The listing builds one solid part. Answer for the finished solid, in the listing's coordinates (mm). A direction names the side the tool comes from. Give positions to 0.01 mm unless a question says otherwise; leave off trailing zeros. Write each loop counter-clockwise with the first axis right and the second up, starting at its lowest first coordinate (ties: lowest second). Pieces come first, ordered by that corner, then holes. Notation, with made-up numbers: M 61.25,26 L 100.25,26 A22 ccw 100.25,62 Z; hole C -26.5,-36.5 d8. An arc over 180 degrees is marked long. Return JSON: item names as keys, results as strings.
from build123d import *

# Parameters (mm, degrees)
SKETCH1_R               = 2.25
BOSS_EXTRUDE1_DEPTH     = 7.5
CUT_EXTRUDE1_START      = 7.5
SKETCH1_3_R             = 6.52
CUT_EXTRUDE1_DEPTH      = 5
CUT_EXTRUDE2_START      = -7.5
SKETCH1_4_R             = 6.52
CUT_EXTRUDE2_DEPTH      = 5
SKETCH2_R               = 14.4
BOSS_EXTRUDE2_DEPTH     = 19
CUT_EXTRUDE3_DEPTH      = 51.395634732
CUT_EXTRUDE3_DEPTH_BACK = 51.395634732
CUT_EXTRUDE4_DEPTH      = 7
CUT_EXTRUDE5_START      = -12
SKETCH2_5_R             = 11.4
CUT_EXTRUDE5_DEPTH      = 7
FILLET1_R               = 5
FILLET2_R               = 10
FILLET3_R               = 5


with BuildPart() as part:
    # Sketch1 → Boss-Extrude1 (new, symmetric)
    with BuildSketch(Plane.XY):
        Polygon((-9.5, 9), (9.5, 9), (9.5, -10.52), (-5.5, -25.52), (-30, -25.52), (-30, -6.52), (-9.5, -6.52), align=None)
        Circle(SKETCH1_R, mode=Mode.SUBTRACT)
    extrude(amount=BOSS_EXTRUDE1_DEPTH, both=True)

    # Sketch1<3> → Cut-Extrude1 (cut)
    with BuildSketch(Plane.XY.offset(CUT_EXTRUDE1_START)):
        Circle(SKETCH1_3_R)
    extrude(amount=-CUT_EXTRUDE1_DEPTH, mode=Mode.SUBTRACT)

    # Sketch1<4> → Cut-Extrude2 (cut)
    with BuildSketch(Plane.XY.offset(CUT_EXTRUDE2_START)):
        Circle(SKETCH1_4_R)
    extrude(amount=CUT_EXTRUDE2_DEPTH, mode=Mode.SUBTRACT)

    # Sketch2 → Boss-Extrude2 (add, through all)
    with BuildSketch(Plane(origin=(0, -6.52, 0), x_dir=(1, 0, 0), z_dir=(0, 1, 0))):
        with Locations((-30, 0)):
            Circle(SKETCH2_R)
    extrude(amount=-BOSS_EXTRUDE2_DEPTH)

    # Sketch2<3> → Cut-Extrude3 (cut, two sides: drawn at the far end of the back side and taken through both)
    with BuildSketch(Plane(origin=(0, -6.52, 0), x_dir=(1, 0, 0), z_dir=(0, 1, 0)).offset(-CUT_EXTRUDE3_DEPTH_BACK)):
        with BuildLine():
            ThreePointArc((-30, -4.25), (-26.99479618, -3.00520382), (-25.75, 0))
            ThreePointArc((-25.75, 0), (-26.99479618, 3.00520382), (-30, 4.25))
            Line((-30, 4.25), (-30, -4.25))
        make_face()
        with BuildLine():
            Line((-30, -4.25), (-30, 4.25))
            ThreePointArc((-30, 4.25), (-34.25, 0), (-30, -4.25))
        make_face()
    extrude(amount=CUT_EXTRUDE3_DEPTH + CUT_EXTRUDE3_DEPTH_BACK, mode=Mode.SUBTRACT)

    # Sketch2<4> → Cut-Extrude4 (cut)
    with BuildSketch(Plane(origin=(0, -6.52, 0), x_dir=(1, 0, 0), z_dir=(0, 1, 0))):
        with BuildLine():
            ThreePointArc((-21.414547187, -7.5), (-19.326805491, -4.005361278), (-18.6, 0))
            ThreePointArc((-18.6, 0), (-19.326805491, 4.005361278), (-21.414547187, 7.5))
            Line((-21.414547187, 7.5), (-30, 7.5))
            Line((-30, 7.5), (-30, 4.25))
            ThreePointArc((-30, 4.25), (-26.99479618, 3.00520382), (-25.75, 0))
            ThreePointArc((-25.75, 0), (-26.99479618, -3.00520382), (-30, -4.25))
            Line((-30, -4.25), (-30, -7.5))
            Line((-30, -7.5), (-21.414547187, -7.5))
        make_face()
        with BuildLine():
            Line((-30, 7.5), (-21.414547187, 7.5))
            ThreePointArc((-21.414547187, 7.5), (-41.4, 0), (-21.414547187, -7.5))
            Line((-21.414547187, -7.5), (-30, -7.5))
            Line((-30, -7.5), (-30, -4.25))
            ThreePointArc((-30, -4.25), (-34.25, 0), (-30, 4.25))
            Line((-30, 4.25), (-30, 7.5))
        make_face()
    extrude(amount=-CUT_EXTRUDE4_DEPTH, mode=Mode.SUBTRACT)

    # Sketch2<5> → Cut-Extrude5 (cut)
    with BuildSketch(Plane(origin=(0, -6.52, 0), x_dir=(1, 0, 0), z_dir=(0, 1, 0)).offset(CUT_EXTRUDE5_START)):
        with Locations(Location((-30, 0, 0), (0, 0, 270))):
            Circle(SKETCH2_5_R)
    extrude(amount=-CUT_EXTRUDE5_DEPTH, mode=Mode.SUBTRACT)

    # Fillet1
    fillet1_edges = [part.edges().sort_by_distance(p)[0] for p in [
        (-9.5, -6.52, 0),
        (-17.707319251, -16.02, -7.5),
        (-17.707319251, -16.02, 7.5),
    ]]
    fillet(fillet1_edges, radius=FILLET1_R)

    # Fillet2
    # the kernel refuses this fillet: 10 mm, written as the material it takes off along each edge
    with BuildSketch(Plane(origin=(-9.5, 9, -32.5), x_dir=(0, -1, 0), z_dir=(0, 0, 1))) as fillet2_piece_1:
        with BuildLine():
            CenterArc((FILLET2_R, FILLET2_R), FILLET2_R, 180, 90)
            Line((0, FILLET2_R), (0, 0))
            Line((0, 0), (FILLET2_R, 0))
        make_face()
    extrude(amount=65, mode=Mode.SUBTRACT)
    with BuildSketch(Plane(origin=(9.5, 9, 32.5), x_dir=(-1, 0, 0), z_dir=(0, 0, -1))) as fillet2_piece_2:
        with BuildLine():
            CenterArc((FILLET2_R, -FILLET2_R), FILLET2_R, 90, 90)
            Line((0, -FILLET2_R), (0, 0))
            Line((0, 0), (FILLET2_R, 0))
        make_face()
    extrude(amount=65, mode=Mode.SUBTRACT)

    # Fillet3
    fillet3_edges = [part.edges().sort_by_distance(p)[0] for p in [
        (2, -18.02, -7.5),
        (9.5, -10.52, 0),
        (2, -18.02, 7.5),
    ]]
    fillet(fillet3_edges, radius=FILLET3_R)


solid = part.part
Item 1: Find the intervals of material crossed by line 1 (Z direction, x = -30, y = -8); line 2 (X direction, y = -8.5, z = 0); line 3 (Z direction, x = -40.5, y = -9.5), in increasing order.
Geometry results:
{"line 1": "z = -14.4 to -11.4, 11.4 to 14.4", "line 2": "x = -44.4 to -41.4, -18.6 to 9.5", "line 3": "z = -9.85 to -4.44, 4.44 to 9.85"}
Item 2: A cutting plane is placed at A-A, the plane y = 0. Write down the section's boundary in (x, z), plus the area to 3 significant figures.
Geometry results:
{"outline": "M -9.45,-7.5 L -6.52,-7.5 L -6.52,-2.5 L -2.25,-2.5 L -2.25,2.5 L -6.52,2.5 L -6.52,7.5 L -9.45,7.5 Z; M 2.25,-2.5 L 6.52,-2.5 L 6.52,-7.5 L 9.45,-7.5 L 9.45,7.5 L 6.52,7.5 L 6.52,2.5 L 2.25,2.5 Z", "area": "131 mm2"}
Item 3: Determine the mould class of faces 1 (the cylindrical face through (6.67, 5.97, 0.11)), 2 (the cylindrical face through (-44.39, -15.89, -0.49)), 3 (the flat face through (-5, -8, -7.5)), 4 (the cylindrical face through (-18.7, -22, -1.5)) for opening direction X: +X half, -X half, draft (parallel to the pull), parting line (faces both ways), or undercut.
Geometry results:
{"face 1": "+X half", "face 2": "parting line", "face 3": "draft", "face 4": "undercut"}
Item 4: A cutting plane is placed at B-B, the plane z = 1.25. Write down the section's boundary in (x, y), plus the area to 3 significant figures.
Geometry results:
{"outline": "M -44.35,-25.52 L -41.33,-25.52 L -41.33,-18.52 L -34.06,-18.52 L -34.06,-13.52 L -41.33,-13.52 L -41.33,-6.52 L -44.35,-6.52 Z; M -25.94,-18.52 L -18.67,-18.52 L -18.67,-25.52 L -5.5,-25.52 L 8.04,-11.98 A5 ccw 9.5,-8.45 L 9.5,-1 A10 ccw 0,8.99 A10 ccw -9.5,-1 L -9.5,-1.52 A5 cw -14.5,-6.52 L -18.67,-6.52 L -18.67,-13.52 L -25.94,-13.52 Z; hole C 0,0 d4.5", "area": "794 mm2"}
Item 5: Given pin 1 Ø1 at (y, z) = (-12.5, -8.5) entering from +X; pin 2 Ø1 at (y, z) = (-17.5, 11.5) entering from -X; pin 3 Ø7.5 at (x, y) = (-4.5, -7.5) entering from -Z, each flat-ended and moving along its own axis, determine where each tip first touches the part or whether it passes through.
Geometry results:
{"pin 1": "stops at x = -17.34", "pin 2": "stops at x = -39.29", "pin 3": "stops at z = -7.5"}
Item 6: A cutting plane is placed at C-C, the plane x = -27. Write down the section's boundary in (y, z).
Geometry results:
{"outline": "M -25.52,-14.08 L -6.52,-14.08 L -6.52,-11 L -13.52,-11 L -13.52,-3.01 L -18.52,-3.01 L -18.52,-11 L -25.52,-11 Z; M -25.52,11 L -18.52,11 L -18.52,3.01 L -13.52,3.01 L -13.52,11 L -6.52,11 L -6.52,14.08 L -25.52,14.08 Z"}
Item 7: A cutting plane is placed at D-D, the plane x = -35.5. Write down the section's boundary in (y, z).
Geometry results:
{"outline": "M -25.52,-13.31 L -6.52,-13.31 L -6.52,-9.99 L -13.52,-9.99 L -13.52,9.99 L -6.52,9.99 L -6.52,13.31 L -25.52,13.31 L -25.52,9.99 L -18.52,9.99 L -18.52,-9.99 L -25.52,-9.99 Z"}
Item 8: Which of the six approach directions +Z, -Z, +X, -X, +Y, -Y give full straight-line access (tool end or side, diameter ignored) to faces 5 (the flat face through (-18, -6.52, -1)), 6 (the flat face through (3, 0, -2.5)), 7 (the flat face through (9.5, -5, 0)), 8 (the flat face through (3, 0, 2.5)), 9 (the cylindrical face through (1, -17, 6))?
Geometry results:
{"face 5": "+Z, -Z, -X, +Y", "face 6": "-Z", "face 7": "+Z, -Z, +X, +Y, -Y", "face 8": "+Z", "face 9": "+Z, +X, -Y"}
